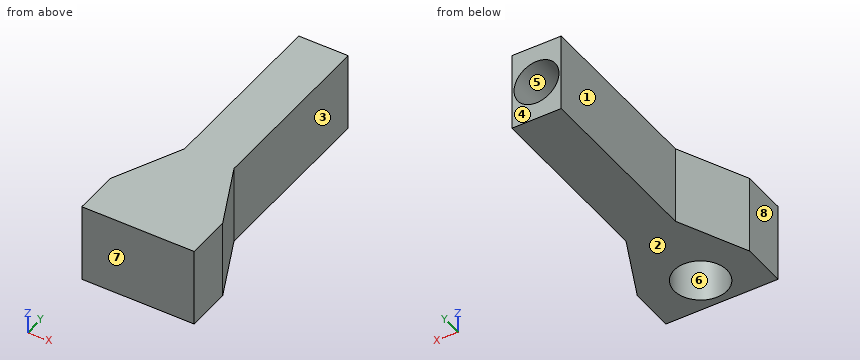
Autodesk Inventor part; units mm, degrees
ref_plane "YZ Plane" through (0, 0, 0) normal (1, 0, 0) x (0, 1, 0)
ref_plane "XZ Plane" through (0, 0, 0) normal (0, 1, 0) x (-1, 0, 0)
ref_plane "XY Plane" through (0, 0, 0) normal (0, 0, 1) x (1, 0, 0)
sketch "Esquisse1" plane through (0, 0, 0) normal (0, 0, 1) x (1, 0, 0)
  line L0 (0, 13) -> (-1.1, 13)
  line L1 (0, 13) -> (1.1, 13)
  line L2 (0, 0) -> (-2.5, 0)
  line L3 (0, 0) -> (2.5, 0)
  line L4 (2.5, 0) -> (2.5, 2)
  line L5 (2.5, 2) -> (1.1, 5)
  line L6 (-2.5, 0) -> (-2.5, 2)
  line L7 (-2.5, 2) -> (-1.1, 5)
  line L8 (-1.1, 5) -> (-1.1, 13)
  line L9 (1.1, 5) -> (1.1, 13)
  dimension "d0" = 13
  dimension "d1" = 1.1
  dimension "d2" = 1.1
  dimension "d3" = 8
  dimension "d5" = 2.5
  dimension "d6" = 2.5
  dimension "d7" = 2
  dimension "d8" = 2
  dimension "d18" = 8
extrude "Extrusion1" add sketch "Esquisse1" along normal blind 3.5
sketch "Esquisse3" plane through (0, 0, 0) normal (0, 0, -1) x (-1, 0, 0)
  line L0 (1.1, 5) -> (2.5, 2)
  line L1 (2.5, 0) -> (-2.5, 0)
  line L2 (2.5, 2) -> (2.5, 0)
  circle A0 centre (0, 1.5) radius 1.175
  line L3 (0, 0) -> (0, 1.5)
  dimension "d14" = 2.35
  dimension "d15" = 1.5
extrude "Extrusion3" cut sketch "Esquisse3" against normal blind 3.3
sketch "Esquisse4" plane through (-1.1, 13, 0) normal (0, 1, 0) x (1, 0, 0)
  line L0 (2.2, 0) -> (2.2, -3.5)
  line L1 (2.2, -1.75) -> (0, -1.75)
  line L2 (0, 0) -> (0, -3.5)
  circle A0 centre (1.1, -1.75) radius 1
  point P0 (1.1, 0)
  dimension "d19" = 2
extrude "Extrusion4" cut sketch "Esquisse4" against normal blind 3
properties part number "Socle P-Barre"
Geometry check sheet. Reference: the model listing, model coordinates, mm. Face numbers are marked on the shaded views. A direction names the side the tool comes from. Give positions to 0.01 mm unless a question says otherwise; leave off trailing zeros. Order: outer loops, then holes, each group sorted by start corner. A loop starts at its lowest first (then second) coordinate and runs counter-clockwise, first axis right, second up. Notation, with made-up numbers: M 3,-5 L 16,-5 A26 ccw 16,26 Z; hole C 52.5,-38.75 d2. An arc over 180 degrees is marked long. Use a Markdown table: item, result.
Item 1: Section check A-A (z = 2.9). Record the cut outline in (x, y) (3 decimals).
Answers follow:
| item | result |
|---|---|
| outline | M -2.5,0 L 2.5,0 L 2.5,2 L 1.1,5 L 1.1,13 L -1.1,13 L -1.1,5 L -2.5,2 Z; hole C 0,1.5 d2.35 |
Item 2: Material ranges on line 1 along Y through (x, z) = (0, 1.2) (3 decimals); line 2 along Z through (x, y) = (0, 10.7); line 3 along X through (y, z) = (1.5, 1.55) (3 decimals), recorded low to high.
Answers follow:
| item | result |
|---|---|
| line 1 | y = 0 to 0.325, 2.675 to 10 |
| line 2 | z = 0 to 0.75, 2.75 to 3.5 |
| line 3 | x = -2.5 to -1.175, 1.175 to 2.5 |
Item 3: Section check D-D (y = 1.5). Record the cut outline in (x, z) (3 decimals).
Answers follow:
| item | result |
|---|---|
| outline | M -2.5,0 L -1.175,0 L -1.175,3.3 L 1.175,3.3 L 1.175,0 L 2.5,0 L 2.5,3.5 L -2.5,3.5 Z |
Item 4: Section check B-B (y = 12). Record the cut outline in (x, z), and give its area (3 significant figures).
Answers follow:
| item | result |
|---|---|
| outline | M -1.1,0 L 1.1,0 L 1.1,3.5 L -1.1,3.5 Z; hole C 0,1.75 d2 |
| area | 4.56 mm2 |
Item 5: Tool access check on the marked faces 1, 2, 3, 4 and 5. Record the directions out of +Z, -Z, +X, -X, +Y, -Y that give a thin tool (end or side, any length) a straight path to the whole face; none if there is none.
Answers follow:
| item | result |
|---|---|
| face 1 | +Z, -Z, -X, +Y |
| face 2 | -Z, +X, -X, +Y, -Y |
| face 3 | +Z, -Z, +X, +Y |
| face 4 | +Z, -Z, +X, -X, +Y |
| face 5 | +Y |
Item 6: Depth check by flat-ended pin: P1, Ø2, axis at y = 11.5, z = 2, coming from the -X side; P2, Ø1, axis at x = 0, y = 6, coming from the -Z side; P3, Ø1.8, axis at y = 10, z = 1, coming from the +X side. Enter the tip coordinate at first touch or a pass-through.
Answers follow:
| item | result |
|---|---|
| P1 | stops at x = -1.1 |
| P2 | stops at z = 0 |
| P3 | stops at x = 1.1 |
Item 7: Section check C-C (x = 0). Record the cut outline in (y, z) (3 decimals).
Answers follow:
| item | result |
|---|---|
| outline | M 0,0 L 0.325,0 L 0.325,3.3 L 2.675,3.3 L 2.675,0 L 13,0 L 13,0.75 L 10,0.75 L 10,2.75 L 13,2.75 L 13,3.5 L 0,3.5 Z |
Item 8: Draft check along X on the marked faces 6, 7 and 8. Enter one of: +X half, -X half, draft (parallel to the pull), parting line (faces both ways), or undercut.
Answers follow:
| item | result |
|---|---|
| face 6 | undercut |
| face 7 | draft |
| face 8 | -X half |
